from build123d import *

# Parameters (mm, degrees)
F0_W     = 20
F0_H     = 40
F1_DEPTH = 4


with BuildPart() as f1:
    # F0 (on Top) → F1 (new body)
    with BuildSketch(Plane.XY):
        with Locations((-1.248105, 5.210561)):
            Rectangle(F0_W, F0_H)
        Polygon((-4.228105, 12.460561), (-4.228105, 9.210561), (1.731895, 9.210561), (1.731895, 12.460561), (2.751895, 12.460561), (2.751895, 9.210561), (6.001895, 9.210561), (6.001895, 8.190561), (2.751895, 8.190561), (2.751895, 2.230561), (6.001895, 2.230561), (6.001895, 1.210561), (2.751895, 1.210561), (2.751895, -2.039439), (1.731895, -2.039439), (1.731895, 1.210561), (-4.228105, 1.210561), (-4.228105, -2.039439), (-5.248105, -2.039439), (-5.248105, 1.210561), (-8.498105, 1.210561), (-8.498105, 2.230561), (-5.248105, 2.230561), (-5.248105, 8.190561), (-8.498105, 8.190561), (-8.498105, 9.210561), (-5.248105, 9.210561), (-5.248105, 12.460561), align=None, mode=Mode.SUBTRACT)
    extrude(amount=F1_DEPTH)


solid = f1.part
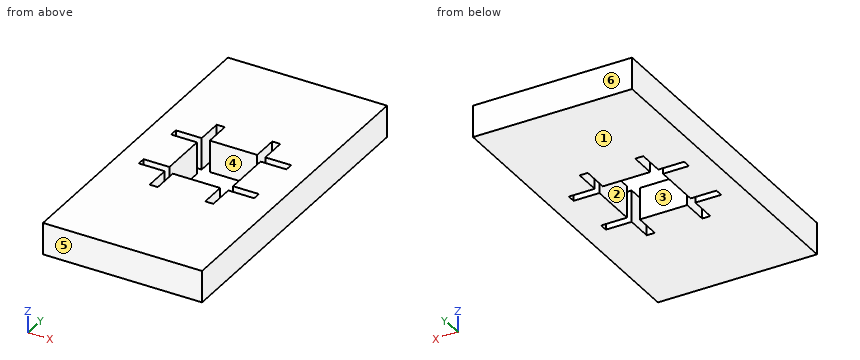
For this review, take the finished solid that the model builds, in its own axes (mm). Face numbers are marked on the shaded views. A direction names the side the tool comes from. Give positions to 0.01 mm unless a question says otherwise; leave off trailing zeros. Order: outer loops, then holes, each group sorted by start corner. A loop starts at its lowest first (then second) coordinate and runs counter-clockwise, first axis right, second up. Notation, with made-up numbers: (43.5, 77.25) -> (83.5, 77.25) arc R26 cw to (83.5, 97.25) -> close; hole circle Ø8 at (-6.75, 23). An arc over 180 degrees is marked (long way). Write item = value, one per line.
1) We need section B-B, the plane x = -2. Give the boundary of the cut face in (y, z), and give its area (3 significant figures).
Findings:
outline = (-14.79, 0) -> (1.21, 0) -> (1.21, 4) -> (-14.79, 4) -> close; (9.21, 0) -> (25.21, 0) -> (25.21, 4) -> (9.21, 4) -> close
area = 128 mm^2
2) We need section C-C, the plane y = 3.5. Give the boundary of the cut face in (x, z), and give its area (3 significant figures).
Findings:
outline = (-11.25, 0) -> (-5.25, 0) -> (-5.25, 4) -> (-11.25, 4) -> close; (2.75, 0) -> (8.75, 0) -> (8.75, 4) -> (2.75, 4) -> close
area = 48.0 mm^2
3) To check wall thickness, follow L1, parallel to Y at x = 4.5, z = 1; L2, parallel to X at y = 0, z = 1.95; L3, parallel to Y at x = -2.5, z = 2.05. State the ranges of each line that lie inside material, in increasing order. Write a range as from..to.
Findings:
L1 = -14.79..1.21, 2.23..8.19, 9.21..25.21
L2 = -11.25..-5.25, -4.23..1.73, 2.75..8.75
L3 = -14.79..1.21, 9.21..25.21
4) Draft analysis for pull direction Y (two halves, no side actions). For the marked faces 3, 4, 5 and 6, state which applies: pulls with the +Y half, pulls with the -Y half, needs draft (parallel to the pull), parting line crosses it, or undercut.
Findings:
face_3 = undercut
face_4 = undercut
face_5 = pulls with the -Y half
face_6 = pulls with the +Y half
5) For the marked faces 1 and 2, list the 3-axis set-ups (+Z, -Z, +X, -X, +Y, -Y) from which the entire face can be reached by the end or side of a thin tool; tool diameter is ignored.
Findings:
face_1 = -Z, +X, -X, +Y, -Y
face_2 = +Z, -Z
